The model under review builds one solid part; all positions refer to its coordinate system, in mm. Face numbers are marked on the shaded views. A direction names the side the tool comes from. Coordinates: 2 decimals unless noted, no trailing zeros. Loops run counter-clockwise (first coordinate to the right, second up) from the corner with the lowest first, then second, coordinate; pieces in that order, holes last. Notation, with made-up numbers: M 19,8.25 L 66,8.25 A9 ccw 66,16.25 Z; hole C -20.5,43.5 d5. An arc over 180 degrees is marked long. Return JSON: item names as keys, results as strings.
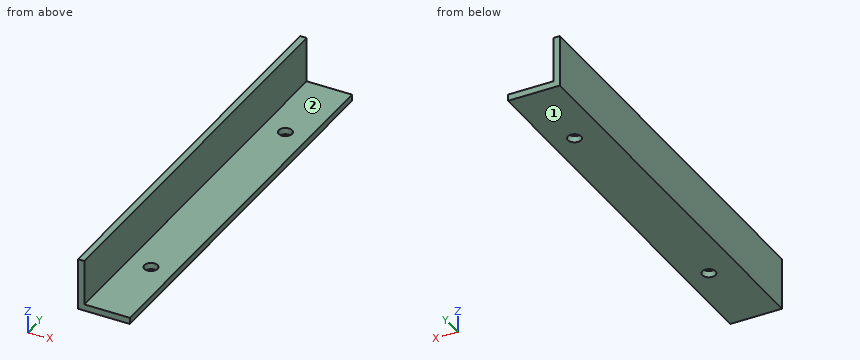
Autodesk Fusion 360 part; units mm, degrees
sketch "Sketch1" plane through (0, 0, 0) normal (0, 1, 0) x (1, 0, 0)
  line L0 (0, -25.4) -> (0, 0)
  line L1 (0, 0) -> (25.4, 0)
  line L2 (12.7, -12.7) -> (11.05, -11.05) construction
  line L3 (3.175, -25.4) -> (3.175, -3.175)
  line L4 (3.175, -3.175) -> (25.4, -3.175)
  line L5 (25.4, -3.175) -> (25.4, 0)
  line L6 (0, -25.4) -> (3.175, -25.4)
  dimension "d1" = 25.4
  dimension "d2" = 25.4
  dimension "d13" = 3.175
extrude "Extrude1" add sketch "Sketch1" along normal blind 100.4
hole "Hole3" at (14.2875, 60.7125, 3.175) direction (0, 0, -1) diameter 6.5 depth 30 tip angle 118
mirror "Mirror2" about plane through (0, 0, 0) normal (0, -1, 0) of bodies 1 merged
equation "d29 = ( 22.225 / 2 ) * 1 mm"
equation "d30 = ( 22.225 / 2 ) * 1 mm + 25.4 mm + 3.175 mm"
1. Insertion check: pin 1 Ø1 at (y, z) = (-60.5, 15.5) entering from -X; pin 2 Ø7.5 at (x, y) = (14.29, -60.71) entering from +Z (3 decimals); pin 3 Ø11 at (y, z) = (16, 17.5) entering from +X (3 decimals); pin 4 Ø2 at (x, z) = (14.5, 4.5) entering from +Y. Each pin has a flat end and moves straight along its axis. Give the tip position at first contact, or say it passes through.
Check values:
{"pin 1": "x = 0", "pin 2": "z = 3.175", "pin 3": "x = 3.175", "pin 4": "through"}
2. Machinability: for the marked faces 1 and 2, which of the approach directions +Z, -Z, +X, -X, +Y, -Y give a long, thin tool a straight path to every point of the face, cutting with its end or side? Answer none if there is none.
Check values:
{"face 1": "-Z, +X, -X, +Y, -Y", "face 2": "+Z, +X, +Y, -Y"}
3. Add section B-B on x = 19.25. Give the boundary of the cut face in (y, z) (3 decimals), plus the area to 3 significant figures.
Check values:
{"outline": "M -100.4,0 L 100.4,0 L 100.4,3.175 L -100.4,3.175 Z", "area": "638 mm²"}
4. To check wall thickness, follow line 1 (X direction, y = -6.5, z = 3.5) (3 decimals). State the ranges of the line that lie inside material, in increasing order.
Check values:
{"line 1": "0 to 3.175"}
5. Add section A-A on y = 61. Give the boundary of the cut face in (x, z) (3 decimals).
Check values:
{"outline": "M 0,0 L 11.05,0 L 11.05,3.175 L 3.175,3.175 L 3.175,25.4 L 0,25.4 Z; M 17.525,0 L 25.4,0 L 25.4,3.175 L 17.525,3.175 Z"}
6. Add section C-C on z = 10.5. Give the boundary of the cut face in (x, y) (3 decimals), plus the area to 3 significant figures.
Check values:
{"outline": "M 0,-100.4 L 3.175,-100.4 L 3.175,100.4 L 0,100.4 Z", "area": "638 mm²"}
